```python
from build123d import *

# Parameters (mm, degrees)
F0_W     = 76.2
F0_H     = 12.7
F1_DEPTH = 6.35
F2_DEPTH = 38.1
F3_R     = 5.08
F4_SIZE  = 1.27
F5_R     = 1.27
F6_R     = 12.7


with BuildPart() as f1:
    # F0 (on Front) → F1 (new body)
    with BuildSketch(Plane.XZ):
        Polygon((-29.878691, -6.35), (-29.878691, 31.75), (-63.618055, 31.75), (-63.618055, -31.75), (-44.521958, -31.75), (-44.521958, -19.05), (-44.521958, -6.35), (-38.028042, -6.35), align=None)
        Polygon((63.618055, -31.75), (63.618055, 31.75), (29.878691, 31.75), (29.878691, -6.35), (38.171958, -6.35), (44.521958, -6.35), (44.521958, -19.05), (44.521958, -31.75), align=None)
        with BuildLine():
            Line((29.878691, -6.35), (29.878691, 31.75))
            Line((29.878691, 31.75), (25.4, 31.75))
            ThreePointArc((25.4, 31.75), (0, 6.35), (-25.4, 31.75))
            Line((-25.4, 31.75), (-29.878691, 31.75))
            Line((-29.878691, 31.75), (-29.878691, -6.35))
            Line((-29.878691, -6.35), (-38.028042, -6.35))
            Line((-38.028042, -6.35), (-44.521958, -6.35))
            Line((-44.521958, -6.35), (-44.521958, -19.05))
            Line((-44.521958, -19.05), (-44.521958, -31.75))
            Line((-44.521958, -31.75), (-38.028042, -31.75))
            Line((-38.028042, -31.75), (-38.028042, -19.05))
            Line((-38.028042, -19.05), (38.171958, -19.05))
            Line((38.171958, -19.05), (38.171958, -31.75))
            Line((38.171958, -31.75), (44.521958, -31.75))
            Line((44.521958, -31.75), (44.521958, -19.05))
            Line((44.521958, -19.05), (44.521958, -6.35))
            Line((44.521958, -6.35), (38.171958, -6.35))
            Line((38.171958, -6.35), (29.878691, -6.35))
        make_face()
        with Locations((0.071958, -25.4)):
            Rectangle(F0_W, F0_H)
    extrude(amount=F1_DEPTH)

    # F0 (on Front) → F2 (join)
    with BuildSketch(Plane.XZ):
        with BuildLine():
            Line((29.878691, -6.35), (29.878691, 31.75))
            Line((29.878691, 31.75), (25.4, 31.75))
            ThreePointArc((25.4, 31.75), (0, 6.35), (-25.4, 31.75))
            Line((-25.4, 31.75), (-29.878691, 31.75))
            Line((-29.878691, 31.75), (-29.878691, -6.35))
            Line((-29.878691, -6.35), (-38.028042, -6.35))
            Line((-38.028042, -6.35), (-44.521958, -6.35))
            Line((-44.521958, -6.35), (-44.521958, -19.05))
            Line((-44.521958, -19.05), (-44.521958, -31.75))
            Line((-44.521958, -31.75), (-38.028042, -31.75))
            Line((-38.028042, -31.75), (-38.028042, -19.05))
            Line((-38.028042, -19.05), (38.171958, -19.05))
            Line((38.171958, -19.05), (38.171958, -31.75))
            Line((38.171958, -31.75), (44.521958, -31.75))
            Line((44.521958, -31.75), (44.521958, -19.05))
            Line((44.521958, -19.05), (44.521958, -6.35))
            Line((44.521958, -6.35), (38.171958, -6.35))
            Line((38.171958, -6.35), (29.878691, -6.35))
        make_face()
    extrude(amount=F2_DEPTH)

    # F3
    f3_edges = [f1.edges().sort_by_distance(p)[0] for p in [
        (-63.618055, -3.175, 31.75),
        (63.618055, -3.175, 31.75),
    ]]
    fillet(f3_edges, radius=F3_R)

    # F4
    f4_edges = [f1.edges().sort_by_distance(p)[0] for p in [
        (0, -38.1, 6.35),
    ]]
    chamfer(f4_edges, length=F4_SIZE)

    # F5
    f5_edges = [f1.edges().sort_by_distance(p)[0] for p in [
        (25.4, -18.415, 31.75),
        (-25.4, -18.415, 31.75),
    ]]
    fillet(f5_edges, radius=F5_R)

    # F6
    f6_edges = [f1.edges().sort_by_distance(p)[0] for p in [
        (-29.878691, -22.225, -6.35),
    ]]
    fillet(f6_edges, radius=F6_R)


solid = f1.part
```
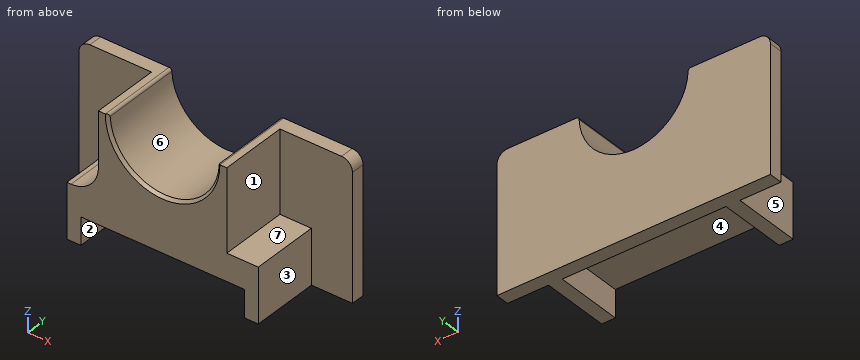
The listing builds one solid part. Answer for the finished solid, in the listing's coordinates (mm). Face numbers are marked on the shaded views. A direction names the side the tool comes from. Give positions to 0.01 mm unless a question says otherwise; leave off trailing zeros. Order: outer loops, then holes, each group sorted by start corner. A loop starts at its lowest first (then second) coordinate and runs counter-clockwise, first axis right, second up. Notation, with made-up numbers: (47, 51) -> (53, 51) arc R8 ccw to (53, 61) -> close; hole circle Ø1 at (36, 48.5). An arc over 180 degrees is marked (long way). Write each question's results on one line, items separated by ' | '.
Q1. Each of these flat-tipped pins is pushed along its axis until it touches: P1, Ø2, axis at y = -28.5, z = -13.5, coming from the +X side; P2, Ø4, axis at x = 9.5, z = -27.5, coming from the -Y side; P3, Ø5, axis at x = -1.5, y = -24, coming from the -Z side. Where does it stop, or does it pass through?
Checked values:
P1: stops at x = 44.52 | P2: stops at y = -6.35 | P3: stops at z = -19.05
Q2. The part is cut by section D-D, the plane z = -24. Give the vertices of the cut face in (x, y), and give its area (3 significant figures).
Checked values:
outline: (-63.62, -6.35) -> (-44.52, -6.35) -> (-44.52, -38.1) -> (-38.03, -38.1) -> (-38.03, -6.35) -> (38.17, -6.35) -> (38.17, -38.1) -> (44.52, -38.1) -> (44.52, -6.35) -> (63.62, -6.35) -> (63.62, 0) -> (-63.62, 0) -> close | area: 1,220 mm^2
Q3. Which of the six approach directions +Z, -Z, +X, -X, +Y, -Y give full straight-line access (tool end or side, diameter ignored) to the marked faces 1, 2 and 3?
Checked values:
face 1: +Z, +X, -Y | face 2: -Z, -Y | face 3: +Z, -Z, +X, -Y
Q4. The part is cut by section C-C, the plane x = 0. Give the vertices of the cut face in (y, z).
Checked values:
outline: (-38.1, -19.05) -> (-6.35, -19.05) -> (-6.35, -31.75) -> (0, -31.75) -> (0, 6.35) -> (-36.83, 6.35) -> (-38.1, 5.08) -> close
Q5. The part is cut by section A-A, the plane y = -17. Give the vertices of the cut face in (x, z), and give its area (3 significant figures).
Checked values:
outline: (-44.52, -31.75) -> (-38.03, -31.75) -> (-38.03, -19.05) -> (38.17, -19.05) -> (38.17, -31.75) -> (44.52, -31.75) -> (44.52, -6.35) -> (29.88, -6.35) -> (29.88, 31.75) -> (26.64, 31.75) arc R1.27 ccw to (25.37, 30.54) arc R25.4 cw to (-25.37, 30.54) arc R1.27 ccw to (-26.64, 31.75) -> (-29.88, 31.75) -> (-29.88, 6.35) arc R12.7 cw to (-42.58, -6.35) -> (-44.52, -6.35) -> close | area: 2,590 mm^2
Q6. Determine the mould class of the marked faces 4, 5, 6 and 7 for opening direction X: pulls with the +X half, pulls with the -X half, needs draft (parallel to the pull), parting line crosses it, or undercut.
Checked values:
face 4: undercut | face 5: pulls with the -X half | face 6: undercut | face 7: needs draft
Q7. Straight lines are drawn through the part: probe 1 along Y at (x, z) = (53.5, -8); probe 2 along Z at (x, y) = (0.5, -4); probe 3 along X at (y, z) = (-18.5, -14.5). For each, find the intervals that lie inside material, in ascending order. Write a range as from..to.
Checked values:
probe 1: y = -6.35..0 | probe 2: z = -31.75..6.35 | probe 3: x = -44.52..44.52
Q8. The part is cut by section B-B, the plane z = -15. Give the vertices of the cut face in (x, y), and give its area (3 significant figures).
Checked values:
outline: (-63.62, -6.35) -> (-44.52, -6.35) -> (-44.52, -38.1) -> (44.52, -38.1) -> (44.52, -6.35) -> (63.62, -6.35) -> (63.62, 0) -> (-63.62, 0) -> close | area: 3,640 mm^2
